Verification items for the finished model (mm, model axes). Coordinates: 2 decimals unless noted, no trailing zeros. Order: outer loops, then holes, each group sorted by start corner. A loop starts at its lowest first (then second) coordinate and runs counter-clockwise, first axis right, second up. Notation, with made-up numbers: (62.25, 84) - (69.25, 84) arc R20 cw to (69.25, 105) - close; hole circle Ø10 at (13, 82). An arc over 180 degrees is marked (long way). Answer as CSV lines item,"result". Start each with the question number.
1. Section check C-C (z = -70). Record the cut outline in (x, y).
2. Section check A-A (x = 93.98). Record the cut outline in (y, z), and give its area (3 significant figures).
3. Go/stop test with flat-tipped pins: pin 1 (1.2 mm diameter, centred on y = 3.5, z = -65, fed in from +X); pin 2 (1.2 mm diameter, centred on x = 64.5, y = 3, fed in from +Z); pin 3 (1.5 mm diameter, centred on y = 4.5, z = -84.5, fed in from -X); pin 4 (1.5 mm diameter, centred on x = 32, z = -68.5, fed in from -Y). Record where each tip stops, or that it passes through.
4. Mould release check, pull along Z, two halves, no side actions. Record for faces 1 (the cylindrical face through (96.253, 2.962, -46.186)), 2 (the flat face through (63, 5.842, -53)), 3 (the cylindrical face through (52.488, 2.88, -13.908)): pulls with the +Z half, pulls with the -Z half, needs draft (parallel to the pull), parting line crosses it, or undercut.
5. Section check B-B (y = 2.35). Record the cut outline in (x, z) (1 decimal).
6. Material ranges on L1, parallel to Z at x = 93.98, y = 1.5; L2, parallel to Z at x = 106, y = 4.9; L3, parallel to X at y = 2.4, z = -98, recorded low to high. Write a range as [from, to].
7. Section check D-D (z = -43.5). Record the cut outline in (x, y).
from build123d import *

# Parameters (mm, degrees)
SKETCH6_R           = 50.8
BOSS_EXTRUDE3_DEPTH = 5.842
CUT_EXTRUDE2_DEPTH  = 6.842
SKETCH12_R          = 2.75
CUT_EXTRUDE3_DEPTH  = 6.842
SKETCH12_3_R        = 2.75
BOSS_EXTRUDE4_DEPTH = 5.842


with BuildPart() as part:
    # Sketch6 → Boss-Extrude3 (new body)
    with BuildSketch(Plane(origin=(0, 0, 0), x_dir=(1, 0, 0), z_dir=(0, 1, 0))):
        with Locations((63.5, 63.5)):
            Circle(SKETCH6_R)
    extrude(amount=BOSS_EXTRUDE3_DEPTH)

    # Sketch11 → Cut-Extrude2 (cut, through all)
    with BuildSketch(Plane(origin=(0, 5.842, 0), x_dir=(1, 0, 0), z_dir=(0, 1, 0))):
        with BuildLine():
            ThreePointArc((80.9625, 93.98), (75.847852166, 106.327852166), (63.5, 111.4425))
            Line((63.5, 111.4425), (63.5, 76.5175))
            ThreePointArc((63.5, 76.5175), (75.847852166, 81.632147834), (80.9625, 93.98))
        make_face()
        with BuildLine():
            Line((63.5, 76.5175), (63.5, 111.4425))
            ThreePointArc((63.5, 111.4425), (46.0375, 93.98), (63.5, 76.5175))
        make_face()
        with BuildLine():
            ThreePointArc((111.4425, 63.5), (93.98, 80.9625), (76.5175, 63.5))
            Line((76.5175, 63.5), (111.4425, 63.5))
        make_face()
        with BuildLine():
            Line((111.4425, 63.5), (76.5175, 63.5))
            ThreePointArc((76.5175, 63.5), (93.98, 46.0375), (111.4425, 63.5))
        make_face()
    extrude(amount=-CUT_EXTRUDE2_DEPTH, mode=Mode.SUBTRACT)

    # Sketch12 → Cut-Extrude3 (cut, through all)
    with BuildSketch(Plane(origin=(0, 5.842, 0), x_dir=(1, 0, 0), z_dir=(0, 1, 0))):
        with Locations((63.5, 63.5)):
            Circle(SKETCH12_R)
    extrude(amount=-CUT_EXTRUDE3_DEPTH, mode=Mode.SUBTRACT)

    # Sketch12<3> → Boss-Extrude4 (add)
    with BuildSketch(Plane(origin=(0, 5.842, 0), x_dir=(1, 0, 0), z_dir=(0, 1, 0))):
        with Locations((63.5, 63.5)):
            Circle(SKETCH12_3_R)
        with BuildLine():
            Line((62.7, 64.23137085), (62.7, 65.69411255))
            ThreePointArc((62.7, 65.69411255), (63.5, 65.820249175), (64.3, 65.69411255))
            Line((64.3, 65.69411255), (64.3, 64.23137085))
            Line((64.3, 64.23137085), (65.7627417, 64.23137085))
            ThreePointArc((65.7627417, 64.23137085), (65.867727335, 63.5), (65.7627417, 62.76862915))
            Line((65.7627417, 62.76862915), (64.3, 62.76862915))
            Line((64.3, 62.76862915), (64.3, 61.30588745))
            ThreePointArc((64.3, 61.30588745), (63.5, 61.179750825), (62.7, 61.30588745))
            Line((62.7, 61.30588745), (62.7, 62.76862915))
            Line((62.7, 62.76862915), (61.2372583, 62.76862915))
            ThreePointArc((61.2372583, 62.76862915), (61.132272665, 63.5), (61.2372583, 64.23137085))
            Line((61.2372583, 64.23137085), (62.7, 64.23137085))
        make_face(mode=Mode.SUBTRACT)
    extrude(amount=-BOSS_EXTRUDE4_DEPTH)


solid = part.part
Evaluation:
1,outline,"(13.12, 0) - (77.77, 0) - (77.77, 5.84) - (13.12, 5.84) - close; (110.19, 0) - (113.88, 0) - (113.88, 5.84) - (110.19, 5.84) - close"
2,outline,"(0, -104.14) - (5.84, -104.14) - (5.84, -80.96) - (0, -80.96) - close; (0, -46.04) - (5.84, -46.04) - (5.84, -22.86) - (0, -22.86) - close"
2,area,"271 mm²"
3,pin 1,"stops at x = 114.29"
3,pin 2,"stops at z = -12.7"
3,pin 3,"stops at x = 16.91"
3,pin 4,"stops at y = 0"
4,face 1,"undercut"
4,face 2,"needs draft"
4,face 3,"parting line crosses it"
5,outline,"circle Ø101.6 at (63.5, -63.5); hole circle Ø34.9 at (63.5, -94); hole (61.2, -64.2) - (62.7, -64.2) - (62.7, -65.7) arc R2.6 ccw to (64.3, -65.7) - (64.3, -64.2) - (65.8, -64.2) arc R2.6 ccw to (65.8, -62.8) - (64.3, -62.8) - (64.3, -61.3) arc R2.6 ccw to (62.7, -61.3) - (62.7, -62.8) - (61.2, -62.8) arc R2.6 ccw to start; hole circle Ø34.9 at (94, -63.5)"
6,L1,"z = [-104.14, -80.96], [-46.04, -22.86]"
6,L2,"z = [-91.33, -76.17], [-50.83, -35.67]"
6,L3,"x = [26.21, 46.51], [80.49, 100.79]"
7,outline,"(16.8, 0) - (110.2, 0) - (110.2, 5.84) - (16.8, 5.84) - close"
